The listing builds one solid part. Answer for the finished solid, in the listing's coordinates (mm). Face numbers are marked on the shaded views. A direction names the side the tool comes from. Round coordinates to 2 decimals unless told otherwise and drop trailing zeros. Write each loop counter-clockwise with the first axis right and the second up, starting at its lowest first coordinate (ties: lowest second). Pieces come first, ordered by that corner, then holes. Notation, with made-up numbers: M 19.25,-35.5 L 46.25,-35.5 A16 cw 46.25,-25.5 Z; hole C -14.5,25.5 d2. An arc over 180 degrees is marked long. Put each result on its own line as item: value. Start each with the question number.
```python
from build123d import *

# Parameters (mm, degrees)
SALIENTE_EXTRUIR1_DEPTH = 10
CROQUIS9_R              = 1.9
CORTAR_EXTRUIR5_DEPTH   = 60.926705232
CORTAR_EXTRUIR6_DEPTH   = 2.75
CROQUIS11_W             = 77.8
CROQUIS11_H             = 1.5
SALIENTE_EXTRUIR2_DEPTH = 0.2
CORTAR_EXTRUIR7_DEPTH   = 2.5
CROQUIS13_R             = 1.8
CORTAR_EXTRUIR8_DEPTH   = 59.728102302


with BuildPart() as part:
    # Croquis1 → Saliente-Extruir1 (new body)
    with BuildSketch(Plane.XY):
        with BuildLine():
            Line((51.5, 9.3), (-51.5, 9.3))
            ThreePointArc((-51.5, 9.3), (-55.742640687, 7.542640687), (-57.5, 3.3))
            Line((-57.5, 3.3), (-57.5, -3.3))
            ThreePointArc((-57.5, -3.3), (-55.742640687, -7.542640687), (-51.5, -9.3))
            Line((-51.5, -9.3), (-44.9, -9.3))
            ThreePointArc((-44.9, -9.3), (-40.657359313, -7.542640687), (-38.9, -3.3))
            Line((-38.9, -3.3), (-38.9, -1.5))
            Line((-38.9, -1.5), (-44.276990951, -1.5))
            ThreePointArc((-44.276990951, -1.5), (-51.659768778, -2.38117618), (-48.2, 4.2))
            Line((-48.2, 4.2), (-38.9, 4.2))
            Line((-38.9, 4.2), (-38.9, 4.3))
            Line((-38.9, 4.3), (38.9, 4.3))
            Line((38.9, 4.3), (38.9, 4.2))
            Line((38.9, 4.2), (48.2, 4.2))
            ThreePointArc((48.2, 4.2), (51.169848481, 2.969848481), (52.4, 0))
            ThreePointArc((52.4, 0), (48.96268014, -4.130171789), (44.276990951, -1.5))
            Line((44.276990951, -1.5), (38.9, -1.5))
            Line((38.9, -1.5), (38.9, -3.3))
            ThreePointArc((38.9, -3.3), (40.657359313, -7.542640687), (44.9, -9.3))
            Line((44.9, -9.3), (51.5, -9.3))
            ThreePointArc((51.5, -9.3), (55.742640687, -7.542640687), (57.5, -3.3))
            Line((57.5, -3.3), (57.5, 3.3))
            ThreePointArc((57.5, 3.3), (55.742640687, 7.542640687), (51.5, 9.3))
        make_face()
    extrude(amount=SALIENTE_EXTRUIR1_DEPTH)

    # Croquis9 → Cortar-Extruir5 (cut, through all)
    with BuildSketch(Plane(origin=(0, 4.3, 0), x_dir=(-1, 0, 0), z_dir=(0, -1, 0))):
        with Locations(Location((0, -5.5, 0), (0, 0, 90))):
            Circle(CROQUIS9_R)
        with Locations(Location((-29.498076211, -5.5, 0), (0, 0, 90))):
            Circle(CROQUIS9_R)
        with Locations(Location((-14.748076211, -5.5, 0), (0, 0, 90))):
            Circle(CROQUIS9_R)
        with Locations(Location((14.748076211, -5.5, 0), (0, 0, 90))):
            Circle(CROQUIS9_R)
        with Locations(Location((29.498076211, -5.5, 0), (0, 0, 90))):
            Circle(CROQUIS9_R)
    extrude(amount=-CORTAR_EXTRUIR5_DEPTH, mode=Mode.SUBTRACT)

    # Croquis10 → Cortar-Extruir6 (cut)
    with BuildSketch(Plane.XZ.offset(-9.3)):
        Polygon((1.098358677, 2.275571128), (3.341616654, 4.838992081), (2.243257977, 8.063420953), (-1.098358677, 8.724428872), (-3.341616654, 6.161007919), (-2.243257977, 2.936579047), align=None)
        Polygon((13.649717534, 2.275571128), (16.991334188, 2.936579047), (18.089692866, 6.161007919), (15.846434889, 8.724428872), (12.504818234, 8.063420953), (11.406459557, 4.838992081), align=None)
        Polygon((28.399717534, 2.275571128), (31.741334188, 2.936579047), (32.839692866, 6.161007919), (30.596434889, 8.724428872), (27.254818234, 8.063420953), (26.156459557, 4.838992081), align=None)
        Polygon((-13.649717534, 2.275571128), (-11.406459557, 4.838992081), (-12.504818234, 8.063420953), (-15.846434889, 8.724428872), (-18.089692866, 6.161007919), (-16.991334188, 2.936579047), align=None)
        Polygon((-28.399717534, 2.275571128), (-26.156459557, 4.838992081), (-27.254818234, 8.063420953), (-30.596434889, 8.724428872), (-32.839692866, 6.161007919), (-31.741334188, 2.936579047), align=None)
    extrude(amount=CORTAR_EXTRUIR6_DEPTH, mode=Mode.SUBTRACT)

    # Croquis11 → Saliente-Extruir2 (add)
    with BuildSketch(Plane.XZ.offset(-4.3)):
        with Locations((0, 9.25)):
            Rectangle(CROQUIS11_W, CROQUIS11_H)
    extrude(amount=SALIENTE_EXTRUIR2_DEPTH)

    # Croquis12 → Cortar-Extruir7 (cut)
    with BuildSketch(Plane(origin=(0, 0, 0), x_dir=(-1, 0, 0), z_dir=(0, 0, -1))):
        Polygon((25.589101615, 6.8), (23.857050808, 9.8), (20.392949192, 9.8), (18.660898385, 6.8), (20.392949192, 3.8), (23.857050808, 3.8), align=None)
        Polygon((-18.665898385, 6.8), (-20.397949192, 9.8), (-23.862050808, 9.8), (-25.594101615, 6.8), (-23.862050808, 3.8), (-20.397949192, 3.8), align=None)
    extrude(amount=-CORTAR_EXTRUIR7_DEPTH, mode=Mode.SUBTRACT)

    # Croquis13 → Cortar-Extruir8 (cut, through all)
    with BuildSketch(Plane(origin=(0, 0, 2.5), x_dir=(-1, 0, 0), z_dir=(0, 0, -1))):
        with Locations((22.125, 6.8)):
            Circle(CROQUIS13_R)
        with Locations((-22.13, 6.8)):
            Circle(CROQUIS13_R)
    extrude(amount=-CORTAR_EXTRUIR8_DEPTH, mode=Mode.SUBTRACT)


solid = part.part
```
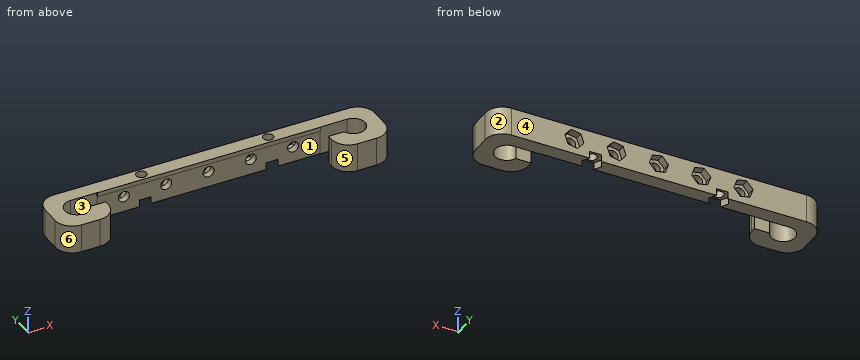
Item 1: Consider line 1 along Y through (x, z) = (12, 0.75); line 2 along X through (y, z) = (-3, 4.75); line 3 along Y through (x, z) = (-21.5, 9.25). Determine where each line is inside the solid, lowest interval first. Write a range as [from, to].
Item 2: Determine the mould class of the marked faces 3, 4, 5 and 6 for opening direction X: released by +X, released by -X, zero draft, split by the parting line, or undercut.
Item 3: Section B-B (x = 0) is taken. Give the vertices of the cut face in (y, z).
Item 4: Section A-A (x = 22.13) is taken. Give the vertices of the cut face in (y, z), and give its area (3 significant figures).
Item 5: Flat-ended cylindrical pins translate along their axes: pin 1 (3 mm diameter, centred on x = 0.5, z = 4, fed in from +Y); pin 2 (10 mm diameter, centred on x = 18, y = -2, fed in from -Z); pin 3 (1 mm diameter, centred on x = 1.5, z = 2, fed in from -Y); pin 4 (1.6 mm diameter, centred on x = 9, z = 9, fed in from -Y). Find the tip coordinate at first contact, or state that the pin passes through.
Item 6: Which of the six approach directions +Z, -Z, +X, -X, +Y, -Y give full straight-line access (tool end or side, diameter ignored) to the marked faces 1 and 2?
Output values:
1. line 1: y = [4.3, 9.3]
1. line 2: x = [-57.5, -51.14], [-45.26, -38.9], [38.9, 45.26], [51.14, 57.5]
1. line 3: y = [4.1, 5.11], [8.49, 9.3]
2. face 3: undercut
2. face 4: zero draft
2. face 5: undercut
2. face 6: released by -X
3. outline: M 4.1,8.5 L 4.3,8.5 L 4.3,7.4 L 6.55,7.4 L 6.55,8.51 L 9.3,8.51 L 9.3,10 L 4.1,10 Z; M 4.3,0 L 9.3,0 L 9.3,2.49 L 6.55,2.49 L 6.55,3.6 L 4.3,3.6 Z
4. outline: M 4.1,8.5 L 4.3,8.5 L 4.3,2.5 L 5,2.5 L 5,10 L 4.1,10 Z; M 8.6,2.5 L 9.3,2.5 L 9.3,10 L 8.6,10 Z
4. area: 10.8 mm^2
5. pin 1: stops at y = 6.55
5. pin 2: passes through
5. pin 3: stops at y = 4.3
5. pin 4: stops at y = 4.1
6. face 1: -Z, -Y
6. face 2: +Z, -Z, +X, +Y
